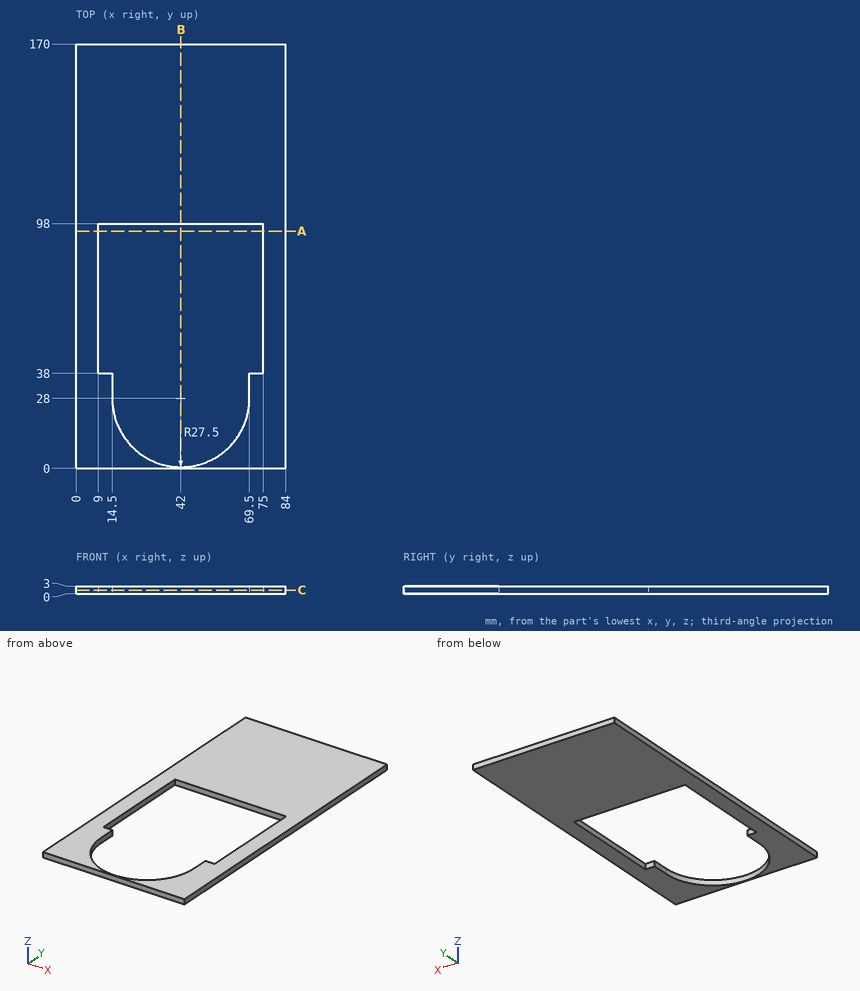
Input: dimensioned drawing with shaded views. Units: mm. Origin: part minimum x, y, z. Coordinates: 2 decimals unless noted, no trailing zeros. Order: outer loops, then holes, each group sorted by start corner. A loop starts at its lowest first (then second) coordinate and runs counter-clockwise, first axis right, second up. Notation, with made-up numbers: (-29.75, -3) - (-13.75, -3) arc R28 cw to (-13.75, 30) - close; hole circle Ø2 at (4, -17.75). An arc over 180 degrees is marked (long way). One line per item, written item: value.
1) Cut plane C-C on z = 1.45. Output: boundary loops of the cut face in (x, y).
Computed values:
outline: (0, 0) - (84, 0) - (84, 170) - (0, 170) - close; hole (9, 38) - (14.5, 38) - (14.5, 28) arc R27.5 ccw to (69.5, 28) - (69.5, 38) - (75, 38) - (75, 98) - (9, 98) - close
2) Cut plane A-A on y = 95. Output: boundary loops of the cut face in (x, z), plus the area to 3 significant figures.
Computed values:
outline: (0, 0) - (9, 0) - (9, 3) - (0, 3) - close; (75, 0) - (84, 0) - (84, 3) - (75, 3) - close
area: 54.0 mm^2
3) Ray query, line 1 (X direction, y = 39, z = 1.55); line 2 (Y direction, x = 53.5, z = 1.9); line 3 (Y direction, x = 66, z = 2.7). Return the intervals inside material, ascending. Write a range as [from, to].
Computed values:
line 1: x = [0, 9], [75, 84]
line 2: y = [0, 3.02], [98, 170]
line 3: y = [0, 14.57], [98, 170]
4) Cut plane B-B on x = 42. Output: boundary loops of the cut face in (y, z), plus the area to 4 significant figures.
Computed values:
outline: (0, 0) - (0.5, 0) - (0.5, 3) - (0, 3) - close; (98, 0) - (170, 0) - (170, 3) - (98, 3) - close
area: 217.5 mm^2
